Read the model definition and answer for the solid it produces. Units are mm, in the model's axes. A direction names the side the tool comes from. Coordinates: 2 decimals unless noted, no trailing zeros. Order: outer loops, then holes, each group sorted by start corner. A loop starts at its lowest first (then second) coordinate and runs counter-clockwise, first axis right, second up. Notation, with made-up numbers: M -15.5,15.5 L 35.5,15.5 A15 cw 35.5,40.5 Z; hole C 26.25,10 d5. An arc over 180 degrees is marked long. One line per question, with ' | ' between items. Start each with the question number.
1) Find section C-C, the plane y = 6.5. Write down the section's boundary in (x, z), plus the area to 3 significant figures.
2) Find section B-B, the plane z = 102.5. Write down the section's boundary in (x, y), plus the area to 3 significant figures.
3) Given P1, Ø2, axis at x = 1.5, z = 74, coming from the +Y side, flat-ended and moving along its own axis, determine where the tip first touches the part or whether it passes through.
4) Find section A-A, the plane x = 13. Write down the section's boundary in (y, z), plus the area to 3 significant figures.
5) Find section D-D, the plane y = -6. Write down the section's boundary in (x, z), plus the area to 3 significant figures.
6) The mould has two halves that part along X. Classify faces 6 (the face through (0, 34, 68)), 7 (the face through (3, 7, 47.314)), 8 (the face through (28, 53, 29.552)): +X half, -X half, draft (parallel to the pull), parting line (faces both ways), or undercut.
7) A tool of negligible diameter and unlimited length cuts with its end or side. For faces 1 (the face through (30, 47.026, 70)), 2 (the face through (1, 15, 98.159)), 3 (the face through (29, 53, 106.616)), 4 (the face through (29, 20, 26.185)), 5 (the face through (28, 53, 105.03)), from which of +Z, -Z, +X, -X, +Y, -Y can it reach the whole face along a straight path? Write none if from no direction.
8) Consider probe 1 along X at (y, z) = (40, 71.5); probe 2 along Z at (x, y) = (34, -3.5); probe 3 along Y at (x, z) = (40.5, 42.5). Determine where each line is inside the solid, lowest interval first.
from build123d import *

# Parameters (mm, degrees)
SKETCH1_W           = 82.927984002
SKETCH1_H           = 63.220938657
BOSS_EXTRUDE1_DEPTH = 2
SKETCH2_W           = 82.927984002
SKETCH2_H           = 3.465808433
BOSS_EXTRUDE2_DEPTH = 55
SKETCH3_W           = 82.927984002
SKETCH3_H           = 3.967313271
BOSS_EXTRUDE3_DEPTH = 55
SKETCH4_W           = 4.221872701
SKETCH4_H           = 55.787816953
BOSS_EXTRUDE4_DEPTH = 55
SKETCH5_W           = 55
SKETCH5_H           = 3.935807591
BOSS_EXTRUDE5_DEPTH = 59
SKETCH6_W           = 41.500434797
SKETCH6_H           = 30.602093287
CUT_EXTRUDE1_DEPTH  = 59
SKETCH7_W           = 44.576665198
SKETCH7_H           = 66.696896342
BOSS_EXTRUDE6_DEPTH = 1.00351002
SKETCH8_W           = 10.465984431
SKETCH8_H           = 14.175880316
BOSS_EXTRUDE7_DEPTH = 2.561499725
BOSS_EXTRUDE8_DEPTH = 3
SKETCH13_W          = 82.927984002
SKETCH13_H          = 63.220938657
BOSS_EXTRUDE9_DEPTH = 1


with BuildPart() as part:
    # Sketch1 → Boss-Extrude1 (new body)
    with BuildSketch(Plane(origin=(0, 0, 0), x_dir=(0, 0, -1), z_dir=(1, 0, 0))):
        with Locations((-67.649308223, 19.885127524)):
            Rectangle(SKETCH1_W, SKETCH1_H)
    extrude(amount=BOSS_EXTRUDE1_DEPTH)

    # Sketch2 → Boss-Extrude2 (add)
    with BuildSketch(Plane(origin=(2, 0, 0), x_dir=(0, 0, -1), z_dir=(1, 0, 0))):
        with Locations((-67.649308223, 49.762692636)):
            Rectangle(SKETCH2_W, SKETCH2_H)
    extrude(amount=BOSS_EXTRUDE2_DEPTH)

    # Sketch3 → Boss-Extrude3 (add)
    with BuildSketch(Plane(origin=(2, 0, 0), x_dir=(0, 0, -1), z_dir=(1, 0, 0))):
        with Locations((-67.649308223, -9.74168517)):
            Rectangle(SKETCH3_W, SKETCH3_H)
    extrude(amount=BOSS_EXTRUDE3_DEPTH)

    # Sketch4 → Boss-Extrude4 (add)
    with BuildSketch(Plane(origin=(2, 0, 0), x_dir=(0, 0, -1), z_dir=(1, 0, 0))):
        with Locations((-107.002363874, 20.135879943)):
            Rectangle(SKETCH4_W, SKETCH4_H)
    extrude(amount=BOSS_EXTRUDE4_DEPTH)

    # Sketch5 → Boss-Extrude5 (add)
    with BuildSketch(Plane(origin=(0, 48.029788419, 0), x_dir=(-1, 0, 0), z_dir=(0, -1, 0))):
        with Locations((-29.5, -28.153220018)):
            Rectangle(SKETCH5_W, SKETCH5_H)
    extrude(amount=BOSS_EXTRUDE5_DEPTH)

    # Sketch6 → Cut-Extrude1 (cut)
    with BuildSketch(Plane.ZY):
        with Locations((77.408781478, 14.741773436)):
            Rectangle(SKETCH6_W, SKETCH6_H)
    extrude(amount=-CUT_EXTRUDE1_DEPTH, mode=Mode.SUBTRACT)

    # Sketch7 → Boss-Extrude6 (add)
    with BuildSketch(Plane(origin=(0, 48.029788419, -1.234575524), x_dir=(-1, 0, 0), z_dir=(0, -1, 0))):
        with Locations((-29.385955108, -71.399525652)):
            Rectangle(SKETCH7_W, SKETCH7_H)
    extrude(amount=BOSS_EXTRUDE6_DEPTH)

    # Sketch8 → Boss-Extrude7 (add)
    with BuildSketch(Plane(origin=(2, 0, -3.365196523), x_dir=(0, 0, -1), z_dir=(1, 0, 0))):
        with Locations((-45.445727025, 7.087940158)):
            Rectangle(SKETCH8_W, SKETCH8_H)
    extrude(amount=BOSS_EXTRUDE7_DEPTH)

    # Sketch9 → Boss-Extrude8 (add)
    with BuildSketch(Plane(origin=(0, 51.495596852, 0), x_dir=(1, 0, 0), z_dir=(0, 1, 0))):
        with BuildLine():
            Line((1.887912496, -105.030139818), (55.50324265, -105.030139818))
            ThreePointArc((55.50324265, -105.030139818), (56.295978023, -105.822875191), (55.50324265, -106.615610564))
            Line((55.50324265, -106.615610564), (1.887912496, -106.615610564))
            ThreePointArc((1.887912496, -106.615610564), (1.095177123, -105.822875191), (1.887912496, -105.030139818))
        make_face()
        with BuildLine():
            Line((1.206362126, -27.966631884), (54.82169228, -27.966631884))
            ThreePointArc((54.82169228, -27.966631884), (55.614427653, -28.759367257), (54.82169228, -29.552102629))
            Line((54.82169228, -29.552102629), (1.206362126, -29.552102629))
            ThreePointArc((1.206362126, -29.552102629), (0.413626753, -28.759367257), (1.206362126, -27.966631884))
        make_face()
    extrude(amount=BOSS_EXTRUDE8_DEPTH)

    # Sketch13 → Boss-Extrude9 (add)
    with BuildSketch(Plane(origin=(57, 0, 0), x_dir=(0, 0, -1), z_dir=(1, 0, 0))):
        with Locations((-67.649308223, 19.885127524)):
            Rectangle(SKETCH13_W, SKETCH13_H)
    extrude(amount=-BOSS_EXTRUDE9_DEPTH)


solid = part.part
Report:
1) outline: M 0,26.19 L 57,26.19 L 57,109.11 L 0,109.11 L 0,98.16 L 2,98.16 L 2,104.89 L 56,104.89 L 56,30.12 L 2,30.12 L 2,36.85 L 4.56,36.85 L 4.56,47.31 L 2,47.31 L 2,56.66 L 0,56.66 Z | area: 633 mm^2
2) outline: M 0,-11.73 L 57,-11.73 L 57,51.5 L 0,51.5 Z; hole M 2,-7.76 L 56,-7.76 L 56,48.03 L 51.67,48.03 L 51.67,47.03 L 7.1,47.03 L 7.1,48.03 L 2,48.03 Z | area: 636 mm^2
3) P1: stops at y = 51.5
4) outline: M -11.73,26.19 L 51.5,26.19 L 51.5,27.97 L 54.5,27.97 L 54.5,29.55 L 51.5,29.55 L 51.5,105.03 L 54.5,105.03 L 54.5,106.62 L 51.5,106.62 L 51.5,109.11 L -11.73,109.11 Z; hole M -7.76,30.12 L 48.03,30.12 L 48.03,36.82 L 47.03,36.82 L 47.03,103.51 L 48.03,103.51 L 48.03,104.89 L -7.76,104.89 Z | area: 1,150 mm^2
5) outline: M 0,26.19 L 57,26.19 L 57,109.11 L 0,109.11 Z; hole M 2,30.12 L 56,30.12 L 56,104.89 L 2,104.89 Z | area: 689 mm^2
6) face 6: -X half | face 7: undercut | face 8: draft
7) face 1: none | face 2: -X | face 3: +Z, +X, -X, +Y | face 4: -Z, +X, -X, +Y, -Y | face 5: +X, -X, +Y
8) probe 1: x = 0 to 2, 56 to 57 | probe 2: z = 26.19 to 30.12, 104.89 to 109.11 | probe 3: y = -11.73 to -7.76, 47.03 to 51.5
